Answer from the drawing. Dimensions are ordinates in mm from the lowest x, y and z of the part. A direction names the side the tool comes from. Round coordinates to 2 decimals unless told otherwise and drop trailing zeros. Write each loop counter-clockwise with the first axis right and the second up, starting at its lowest first coordinate (ties: lowest second). Pieces come first, ordered by that corner, then holes. Notation, with made-up numbers: (-37.75, 72.25) - (12.25, 72.25) arc R13 ccw to (12.25, 97.25) - close; hole circle Ø11 at (-14.75, 68). An arc over 180 degrees is marked (long way). Answer as CSV lines item,"result". Start each with the question number.
1) Find section C-C on x = 71. Determine the outline of the cut face in (y, z) (1 decimal).
2) Which of the six approach directions +Z, -Z, +X, -X, +Y, -Y give full straight-line access (tool end or side, diameter ignored) to the marked faces 4 and 5?
3) Consider line 1 along Z through (x, y) = (50.8, 22.5) (1 decimal); line 2 along Y through (x, z) = (15.5, 53); line 3 along Z through (x, y) = (50.8, 5.5). Determine where each line is inside the solid, lowest interval first.
4) Each of these flat-tipped pins is pushed along its axis until it touches: pin 1 (6 mm diameter, centred on y = 19, z = 29, fed in from +X); pin 2 (7.5 mm diameter, centred on x = 26.05, z = 36.51, fed in from +Y); pin 3 (10 mm diameter, centred on y = 11, z = 77.5, fed in from -X); pin 4 (2 mm diameter, centred on x = 77.5, y = 11, fed in from -Z). Where does it stop, or does it pass through?
5) For a pull along Z with two mould halves and no side action, classify the marked faces 1, 2 and 3 as +Z half, -Z half, draft (parallel to the pull), parting line (faces both ways), or undercut.
6) Find section B-B on x = 50.8. State how many separate pieces and enclosed holes the cut face has, then the cut area to 3 significant figures.
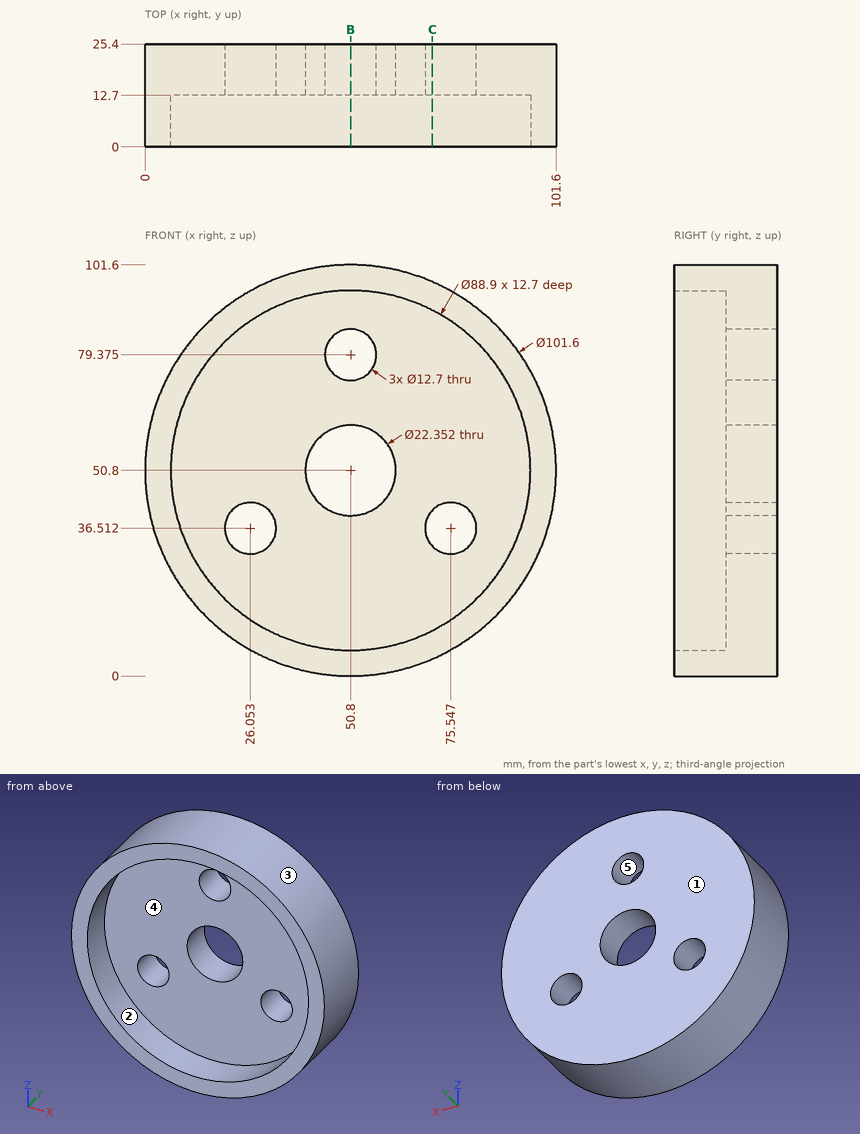
Check values:
1,outline,"(0, 4.2) - (25.4, 4.2) - (25.4, 32.1) - (12.7, 32.1) - (12.7, 11.2) - (0, 11.2) - close; (0, 90.4) - (12.7, 90.4) - (12.7, 40.9) - (25.4, 40.9) - (25.4, 97.4) - (0, 97.4) - close"
2,face 4,"-Y"
2,face 5,"+Y, -Y"
3,line 1,"z = 0 to 39.6, 62 to 73, 85.7 to 101.6"
3,line 2,"y = 12.7 to 25.4"
3,line 3,"z = 0 to 6.35, 95.25 to 101.6"
4,pin 1,"stops at x = 97.99"
4,pin 2,"passes through"
4,pin 3,"stops at x = 4.87"
4,pin 4,"stops at z = 6.98"
5,face 1,"draft"
5,face 2,"undercut"
5,face 3,"parting line"
6,separate pieces,"3"
6,enclosed holes,"0"
6,area,"1,010 mm^2"
